Check sheet for the modelled part. Datum: model origin and axes. Units: mm. Face numbers are marked on the shaded views. A direction names the side the tool comes from. Coordinates: 2 decimals unless noted, no trailing zeros. Write each loop counter-clockwise with the first axis right and the second up, starting at its lowest first coordinate (ties: lowest second). Pieces come first, ordered by that corner, then holes. Notation, with made-up numbers: (0.25, 88.5) -> (51.25, 88.5) arc R15 ccw to (51.25, 113.5) -> close; hole circle Ø11 at (22, 17.5). An arc over 180 degrees is marked (long way). Put each result on its own line as item: value.
```python
from build123d import *

# Parameters (mm, degrees)
SKETCH_1_R          = 48
EXTRUDE_1_DEPTH     = 64
CUT_EXTRUDE_1_DEPTH = 67
EXTRUDE_START       = -56
EXTRUDE_2_DEPTH     = 56
CUT_EXTRUDE_2_DEPTH = 28
SKETCH_5_W          = 44
SKETCH_5_H          = 8
CUT_EXTRUDE_3_DEPTH = 54
SKETCH_6_R          = 28
CUT_EXTRUDE_4_DEPTH = 119.928549979


with BuildPart() as part:
    # 草圖1 → 填料-伸長1 (new body)
    with BuildSketch(Plane(origin=(0, 0, 0), x_dir=(1, 0, 0), z_dir=(0, 1, 0))):
        with Locations(Location((0, 0, 0), (0, 0, 270))):
            Circle(SKETCH_1_R)
    extrude(amount=EXTRUDE_1_DEPTH)

    # 草圖2 → 除料-伸長1 (cut, symmetric)
    with BuildSketch(Plane.XY):
        with BuildLine():
            Line((-48, 38), (12, 38))
            ThreePointArc((12, 38), (18, 32), (12, 26))
            Line((12, 26), (-48, 26))
            Line((-48, 26), (-48, 38))
        make_face()
    extrude(amount=CUT_EXTRUDE_1_DEPTH, both=True, mode=Mode.SUBTRACT)

    # 草圖3 → 填料-伸長2 (add)
    with BuildSketch(Plane(origin=(0, 56, 0), x_dir=(1, 0, 0), z_dir=(0, 1, 0)).offset(EXTRUDE_START)):
        with BuildLine():
            Line((88, -32), (88, 32))
            Line((88, 32), (9.03959037, 47.141126481))
            ThreePointArc((9.03959037, 47.141126481), (48, 0), (9.03959037, -47.141126481))
            Line((9.03959037, -47.141126481), (88, -32))
        make_face()
    extrude(amount=EXTRUDE_2_DEPTH)

    # 草圖4 → 除料-伸長2 (cut)
    with BuildSketch(Plane(origin=(0, 56, 0), x_dir=(1, 0, 0), z_dir=(0, 1, 0))):
        Polygon((88, -16), (88, 16), (78, 16), (78, 20), (56, 20), (56, -20), (78, -20), (78, -16), align=None)
    extrude(amount=-CUT_EXTRUDE_2_DEPTH, mode=Mode.SUBTRACT)

    # 草圖5 → 除料-伸長3 (cut, symmetric)
    with BuildSketch(Plane.XY):
        with Locations((66, 4)):
            Rectangle(SKETCH_5_W, SKETCH_5_H)
    extrude(amount=CUT_EXTRUDE_3_DEPTH, both=True, mode=Mode.SUBTRACT)

    # 草圖6 → 除料-伸長4 (cut, through all)
    with BuildSketch(Plane(origin=(0, 64, 0), x_dir=(1, 0, 0), z_dir=(0, 1, 0))):
        with Locations(Location((0, 0, 0), (0, 0, 270))):
            Circle(SKETCH_6_R)
    extrude(amount=-CUT_EXTRUDE_4_DEPTH, mode=Mode.SUBTRACT)


solid = part.part
```
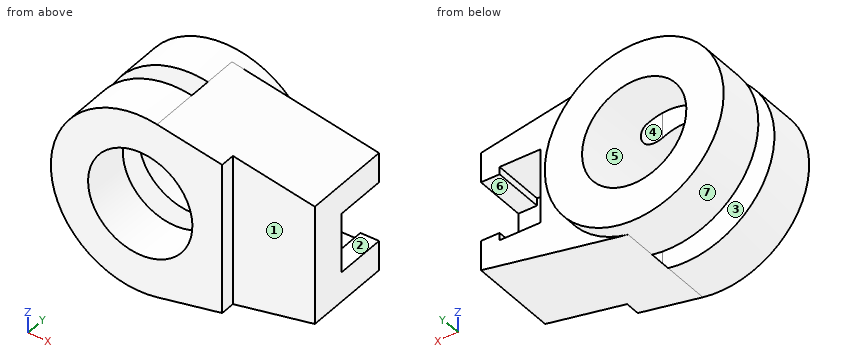
Q1. Cross-section at A-A (z = 0). Record the cut outline in (x, y), plus the area to 3 significant figures.
Recorded:
outline: (-48, 0) -> (-28, 0) -> (-28, 26) -> (-48, 26) -> close; (-48, 38) -> (-28, 38) -> (-28, 64) -> (-48, 64) -> close; (28, 0) -> (44, 0) -> (44, 8) -> (88, 8) -> (88, 28) -> (56, 28) -> (56, 56) -> (48, 56) -> (48, 64) -> (28, 64) -> close
area: 3,310 mm2
Q2. Depth check by flat-ended pin: P1, Ø6, axis at x = 71.5, z = 0.5, coming from the -Y side; P2, Ø1.2, axis at y = 46.5, z = 17.5, coming from the -X side; P3, Ø8, axis at x = 85, y = 38.5, coming from the +Z side. Enter the tip coordinate at first touch or a pass-through.
Recorded:
P1: stops at y = 8
P2: stops at x = -44.93
P3: stops at z = 33.34
Q3. Mould release check, pull along Y, two halves, no side actions. Record for the marked faces 1, 2 and 3: released by +Y, released by -Y, zero draft, split by the parting line, or undercut.
Recorded:
face 1: released by -Y
face 2: zero draft
face 3: undercut
Q4. Cross-section at C-C (x = 0). Record the cut outline in (y, z), plus the area to 3 significant figures.
Recorded:
outline: (0, -48) -> (26, -48) -> (26, -28) -> (0, -28) -> close; (0, 28) -> (26, 28) -> (26, 48) -> (0, 48) -> close; (38, -48) -> (64, -48) -> (64, -28) -> (38, -28) -> close; (38, 28) -> (64, 28) -> (64, 48) -> (38, 48) -> close
area: 2,080 mm2
Q5. Tool access check on the marked faces 4, 5, 6 and 7. Record the directions out of +Z, -Z, +X, -X, +Y, -Y that give a thin tool (end or side, any length) a straight path to the whole face; none if there is none.
Recorded:
face 4: -X
face 5: +Y, -Y
face 6: +X, +Y
face 7: +Y
Q6. Material ranges on line 1 along Y through (x, z) = (8, -31); line 2 along X through (y, z) = (17, 0); line 3 along Z through (x, y) = (0, 13), recorded low to high.
Recorded:
line 1: y = 0 to 26, 38 to 64
line 2: x = -48 to -28, 28 to 88
line 3: z = -48 to -28, 28 to 48
Q7. Cross-section at B-B (y = 50.5). Record the cut outline in (x, z), plus the area to 3 significant figures.
Recorded:
outline: (9.04, -47.14) -> (88, -32) -> (88, -16) -> (78, -16) -> (78, -20) -> (56, -20) -> (56, 20) -> (78, 20) -> (78, 16) -> (88, 16) -> (88, 32) -> (9.04, 47.14) arc R48 ccw (long way) to start; hole circle Ø56 at (0, 0)
area: 7,070 mm2
Q8. Cross-section at D-D (y = 32). Record the cut outline in (x, z).
Recorded:
outline: (9.04, -47.14) -> (88, -32) -> (88, -16) -> (78, -16) -> (78, -20) -> (56, -20) -> (56, 20) -> (78, 20) -> (78, 16) -> (88, 16) -> (88, 32) -> (9.04, 47.14) arc R48 cw to (18, 44.5) -> (18, 21.45) arc R28 cw to (18, -21.45) -> (18, -44.5) arc R48 cw to start
